```python
from build123d import *

# Parameters (mm, degrees)
SKETCH_1_W          = 68
SKETCH_1_H          = 100
EXTRUDE_1_DEPTH     = 1.8
SKETCH_2_W          = 48
SKETCH_2_H          = 5
SKETCH_2_W_2        = 26
SKETCH_2_H_2        = 17
SKETCH_2_W_3        = 3.846350714
SKETCH_2_H_3        = 4
SKETCH_2_W_4        = 50.5
SKETCH_2_H_4        = 25
SKETCH_2_W_5        = 24
SKETCH_2_W_6        = 18
SKETCH_2_H_5        = 16.79174546
SKETCH_2_W_7        = 4.5
SKETCH_2_H_6        = 9
CUT_EXTRUDE_1_DEPTH = 1.8
SKETCH_4_R          = 2.5
SKETCH_4_R_2        = 1.4
SKETCH_4_R_3        = 2
EXTRUDE_3_DEPTH     = 1
CUT_EXTRUDE_START   = -14
SKETCH_6_R          = 1.4
CUT_EXTRUDE_3_DEPTH = 14
SKETCH_8_W          = 5
SKETCH_8_H          = 5
SKETCH_8_W_2        = 18
SKETCH_8_H_2        = 4.20825454
CUT_EXTRUDE_4_DEPTH = 10
SKETCH_9_R          = 1.6
CUT_EXTRUDE_5_DEPTH = 10


with BuildPart() as part:
    # 草图1 → 凸台-拉伸1 (new body)
    with BuildSketch(Plane(origin=(0, 0, 0), x_dir=(1, 0, 0), z_dir=(0, 1, 0))):
        with Locations((34, -50)):
            Rectangle(SKETCH_1_W, SKETCH_1_H)
    extrude(amount=EXTRUDE_1_DEPTH)

    # 草图2 → 切除-拉伸1 (cut)
    with BuildSketch(Plane(origin=(0, 1.8, 0), x_dir=(1, 0, 0), z_dir=(0, 1, 0))):
        with Locations((34, -2.5)):
            Rectangle(SKETCH_2_W, SKETCH_2_H)
        with Locations((34, -23.5)):
            Rectangle(SKETCH_2_W_2, SKETCH_2_H_2)
        with Locations((5.923175357, -26)):
            Rectangle(SKETCH_2_W_3, SKETCH_2_H_3)
        with Locations((5.535050967, -79)):
            Rectangle(SKETCH_2_W_3, SKETCH_2_H_3)
        with Locations((28.75, -57.5)):
            Rectangle(SKETCH_2_W_4, SKETCH_2_H_4)
        with Locations((24, -97.5)):
            Rectangle(SKETCH_2_W_5, SKETCH_2_H)
        with Locations((50, -91.60412727)):
            Rectangle(SKETCH_2_W_6, SKETCH_2_H_5)
        with Locations((59.25, -39.5)):
            Rectangle(SKETCH_2_W_7, SKETCH_2_H_6)
    extrude(amount=-CUT_EXTRUDE_1_DEPTH, mode=Mode.SUBTRACT)

    # 草图4 → 凸台-拉伸3 (add)
    # profile 1 of 4: a face of its own
    with BuildSketch(Plane.XZ):
        with Locations(Location((7, 97, 0), (0, 0, 90))):
            Circle(SKETCH_4_R)
        with Locations(Location((7, 97, 0), (0, 0, 270))):
            Circle(SKETCH_4_R_2, mode=Mode.SUBTRACT)
    # profile 2 of 4: a face of its own
    with BuildSketch(Plane.XZ):
        with Locations(Location((61, 97, 0), (0, 0, 180))):
            Circle(SKETCH_4_R_3)
        with Locations(Location((61, 97, 0), (0, 0, 270))):
            Circle(SKETCH_4_R_2, mode=Mode.SUBTRACT)
    # profile 3 of 4: a face of its own
    with BuildSketch(Plane.XZ):
        with Locations(Location((61, 3, 0), (0, 0, 90))):
            Circle(SKETCH_4_R)
        with Locations(Location((61, 3, 0), (0, 0, 270))):
            Circle(SKETCH_4_R_2, mode=Mode.SUBTRACT)
    # profile 4 of 4: a face of its own
    with BuildSketch(Plane.XZ):
        with Locations(Location((7, 3, 0), (0, 0, 90))):
            Circle(SKETCH_4_R)
        with Locations(Location((7, 3, 0), (0, 0, 270))):
            Circle(SKETCH_4_R_2, mode=Mode.SUBTRACT)
    extrude(amount=EXTRUDE_3_DEPTH)

    # 草图6 → 切除-拉伸3 (cut)
    with BuildSketch(Plane.XZ.offset(CUT_EXTRUDE_START)):
        with Locations(Location((7, 97, 0), (0, 0, 90))):
            Circle(SKETCH_6_R)
        with Locations(Location((61, 97, 0), (0, 0, 90))):
            Circle(SKETCH_6_R)
        with Locations(Location((61, 3, 0), (0, 0, 90))):
            Circle(SKETCH_6_R)
        with Locations(Location((7, 3, 0), (0, 0, 90))):
            Circle(SKETCH_6_R)
    extrude(amount=CUT_EXTRUDE_3_DEPTH, mode=Mode.SUBTRACT)

    # 草图8 → 切除-拉伸4 (cut)
    with BuildSketch(Plane(origin=(0, 1.8, 0), x_dir=(1, 0, 0), z_dir=(0, 1, 0))):
        with Locations((38.5, -97.5)):
            Rectangle(SKETCH_8_W, SKETCH_8_H)
        with Locations((50, -81.10412727)):
            Rectangle(SKETCH_8_W_2, SKETCH_8_H_2)
    extrude(amount=-CUT_EXTRUDE_4_DEPTH, mode=Mode.SUBTRACT)

    # 草图9 → 切除-拉伸5 (cut)
    with BuildSketch(Plane(origin=(0, 1.8, 0), x_dir=(1, 0, 0), z_dir=(0, 1, 0))):
        with Locations(Location((7, -3, 0), (0, 0, 270))):
            Circle(SKETCH_9_R)
        with Locations(Location((61, -3, 0), (0, 0, 270))):
            Circle(SKETCH_9_R)
        with Locations(Location((61, -97, 0), (0, 0, 270))):
            Circle(SKETCH_9_R)
        with Locations(Location((7, -97, 0), (0, 0, 270))):
            Circle(SKETCH_9_R)
    extrude(amount=-CUT_EXTRUDE_5_DEPTH, mode=Mode.SUBTRACT)


solid = part.part
```
For this review, take the finished solid that the model builds, in its own axes (mm). A direction names the side the tool comes from. Round coordinates to 2 decimals unless told otherwise and drop trailing zeros. Order: outer loops, then holes, each group sorted by start corner. A loop starts at its lowest first (then second) coordinate and runs counter-clockwise, first axis right, second up. Notation, with made-up numbers: (-0.5, 64) -> (39.5, 64) arc R24 cw to (39.5, 89) -> close; hole circle Ø1 at (-12.5, -16). An arc over 180 degrees is marked (long way). Use a Markdown table: item, result.
Item 1: Take a section at A-A (y = -0.5). State the section outline as (x, z) points, plus the area to 3 significant figures.
Resolved:
| item | result |
|---|---|
| outline | circle Ø5 at (7, 3); circle Ø5 at (7, 97); circle Ø5 at (61, 3); circle Ø4 at (61, 97); hole circle Ø3.2 at (7, 3); hole circle Ø3.2 at (7, 97); hole circle Ø3.2 at (61, 3); hole circle Ø3.2 at (61, 97) |
| area | 39.3 mm² |
Item 2: For pin 1 (1.4 mm diameter, centred on x = 26, y = 1, fed in from +Z), flat-tipped, find the tip position at first contact; note if it passes through.
Resolved:
| item | result |
|---|---|
| pin 1 | stops at z = 95 |
Item 3: Take a section at B-B (x = 34). State the section outline as (y, z) points, plus the area to 3 significant figures.
Resolved:
| item | result |
|---|---|
| outline | (0, 5) -> (1.8, 5) -> (1.8, 15) -> (0, 15) -> close; (0, 32) -> (1.8, 32) -> (1.8, 45) -> (0, 45) -> close; (0, 70) -> (1.8, 70) -> (1.8, 95) -> (0, 95) -> close |
| area | 86.4 mm² |
Item 4: For line 1 along X through (y, z) = (-0.1, 3); line 2 along X through (y, z) = (0.45, 3); line 3 along X through (y, z) = (1.25, 25.5), list the stretches that pass through material, from the lowest coordinate up. Write a range as [from, to].
Resolved:
| item | result |
|---|---|
| line 1 | x = [4.5, 5.4], [8.6, 9.5], [58.5, 59.4], [62.6, 63.5] |
| line 2 | x = [0, 5.4], [8.6, 10], [58, 59.4], [62.6, 68] |
| line 3 | x = [0, 4], [7.85, 21], [47, 68] |
Item 5: Machinability: for faces 4 (the cylindrical face through (61.26, -0.493, 95.017)), 5 (the cylindrical face through (62.586, 0.42, 2.792)), which of the approach directions +Z, -Z, +X, -X, +Y, -Y give a long, thin tool a straight path to every point of the face, cutting with its end or side? Answer none if there is none.
Resolved:
| item | result |
|---|---|
| face 4 | -Y |
| face 5 | +Y, -Y |
Item 6: Draft analysis for pull direction X (two halves, no side actions). For faces 1 (the cylindrical face through (8.5, -0.5, 1)), 2 (the flat face through (9, -1, 3)), 3 (the cylindrical face through (62.08, 0.42, 95.82)), state which applies: +X half, -X half, draft (parallel to the pull), parting line (faces both ways), or undercut.
Resolved:
| item | result |
|---|---|
| face 1 | undercut |
| face 2 | draft |
| face 3 | undercut |
Item 7: Take a section at D-D (x = 15). State the section outline as (y, z) points, plus the area to 3 significant figures.
Resolved:
| item | result |
|---|---|
| outline | (0, 5) -> (1.8, 5) -> (1.8, 45) -> (0, 45) -> close; (0, 70) -> (1.8, 70) -> (1.8, 95) -> (0, 95) -> close |
| area | 117 mm² |
Item 8: Take a section at C-C (z = 86.5). State the section outline as (x, y) points, plus the area to 3 significant figures.
Resolved:
| item | result |
|---|---|
| outline | (0, 0) -> (41, 0) -> (41, 1.8) -> (0, 1.8) -> close; (59, 0) -> (68, 0) -> (68, 1.8) -> (59, 1.8) -> close |
| area | 90.0 mm² |
